The listing builds one solid part. Answer for the finished solid, in the listing's coordinates (mm). Coordinates: 2 decimals unless noted, no trailing zeros. Order: outer loops, then holes, each group sorted by start corner. A loop starts at its lowest first (then second) coordinate and runs counter-clockwise, first axis right, second up. Notation, with made-up numbers: (30, 76.5) - (69, 76.5) arc R26 cw to (69, 96.5) - close; hole circle Ø6 at (-17.75, -14). An arc over 180 degrees is marked (long way). Use one line per item in the form item = value. Start each with the question number.
Item 1: Consider line 1 along X through (y, z) = (2.4, -47); line 2 along Z through (x, y) = (50, 1.6); line 3 along Z through (x, y) = (59.5, 0.65). Determine where each line is inside the solid, lowest interval first. Write a range as [from, to].
Item 2: Each of these flat-tipped pins is pushed along its axis until it touches: pin 1 Ø1 at (x, y) = (59.5, 1.5) entering from +Z; pin 2 Ø1 at (y, z) = (1.5, -46) entering from +X; pin 3 Ø4.5 at (x, z) = (50.2, 92.2) entering from +Y (3 decimals); pin 4 Ø1.5 at (x, y) = (-71.5, 2) entering from -Z. Where does it stop, or does it pass through?
Item 3: Section C-C, the plane y = 1.6 is taken. Count the separate pieces of the cut face and the enclosed holes in it, and give its area (3 significant figures).
Item 4: Section B-B, the plane z = 51.5 is taken. Write down the section's boundary in (x, y) (3 decimals), and give its area (3 significant figures).
Item 5: Section A-A, the plane x = 0 is taken. Write down the section's boundary in (y, z) (3 decimals), and give its area (3 significant figures).
Item 6: Section D-D, the plane z = 24 is taken. Write down the section's boundary in (x, y) (3 decimals).
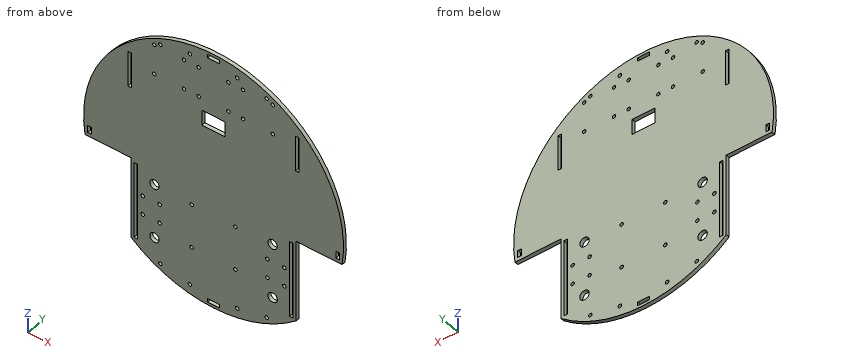
from build123d import *

# Parameters (mm, degrees)
SKETCH_1_R   = 1.5
SKETCH_1_R_2 = 4
SKETCH_1_R_3 = 1.45
SKETCH_1_W   = 10
SKETCH_1_H   = 3
SKETCH_1_W_2 = 19.6
SKETCH_1_H_2 = 12.9
SKETCH_1_W_3 = 3
SKETCH_1_H_3 = 6
SKETCH_1_H_4 = 65
SKETCH_1_H_5 = 30
BASE_DEPTH   = 3.175


with BuildPart() as part:
    # 草图1 → Base (new body)
    with BuildSketch(Plane(origin=(0, 0, 0), x_dir=(1, 0, 0), z_dir=(0, 1, 0))):
        with BuildLine():
            Line((-108.841874295, 15.92), (-70, 15.92))
            Line((-70, 15.92), (-70, 84.852813742))
            ThreePointArc((-70, 84.852813742), (0, 110), (70, 84.852813742))
            Line((70, 84.852813742), (70, 15.92))
            Line((70, 15.92), (108.841874295, 15.92))
            ThreePointArc((108.841874295, 15.92), (0, -110), (-108.841874295, 15.92))
        make_face()
        with Locations((-60, 43.92)):
            Circle(SKETCH_1_R, mode=Mode.SUBTRACT)
        with Locations((-60, 60)):
            Circle(SKETCH_1_R, mode=Mode.SUBTRACT)
        with Locations((-45.65, 60)):
            Circle(SKETCH_1_R, mode=Mode.SUBTRACT)
        with Locations((-45.65, 43.92)):
            Circle(SKETCH_1_R, mode=Mode.SUBTRACT)
        with Locations((60, 60)):
            Circle(SKETCH_1_R, mode=Mode.SUBTRACT)
        with Locations((45.65, 60)):
            Circle(SKETCH_1_R, mode=Mode.SUBTRACT)
        with Locations((45.65, 43.92)):
            Circle(SKETCH_1_R, mode=Mode.SUBTRACT)
        with Locations((60, 43.92)):
            Circle(SKETCH_1_R, mode=Mode.SUBTRACT)
        with Locations((-20, -100)):
            Circle(SKETCH_1_R, mode=Mode.SUBTRACT)
        with Locations((20, -100)):
            Circle(SKETCH_1_R, mode=Mode.SUBTRACT)
        with Locations((20, 100)):
            Circle(SKETCH_1_R, mode=Mode.SUBTRACT)
        with Locations((-20, 100)):
            Circle(SKETCH_1_R, mode=Mode.SUBTRACT)
        with Locations((-50, 75)):
            Circle(SKETCH_1_R_2, mode=Mode.SUBTRACT)
        with Locations((50, 75)):
            Circle(SKETCH_1_R_2, mode=Mode.SUBTRACT)
        with Locations((-18.5, 67)):
            Circle(SKETCH_1_R, mode=Mode.SUBTRACT)
        with Locations((-18.5, 30)):
            Circle(SKETCH_1_R, mode=Mode.SUBTRACT)
        with Locations((18.5, 30)):
            Circle(SKETCH_1_R, mode=Mode.SUBTRACT)
        with Locations((18.5, 67)):
            Circle(SKETCH_1_R, mode=Mode.SUBTRACT)
        with Locations((-12.6, -67)):
            Circle(SKETCH_1_R_3, mode=Mode.SUBTRACT)
        with Locations((-12.6, -92.2)):
            Circle(SKETCH_1_R_3, mode=Mode.SUBTRACT)
        with Locations((12.6, -92.2)):
            Circle(SKETCH_1_R_3, mode=Mode.SUBTRACT)
        with Locations((12.6, -67)):
            Circle(SKETCH_1_R_3, mode=Mode.SUBTRACT)
        with Locations((-45, 95)):
            Circle(SKETCH_1_R, mode=Mode.SUBTRACT)
        with Locations((45, 95)):
            Circle(SKETCH_1_R, mode=Mode.SUBTRACT)
        with Locations((45, -95)):
            Circle(SKETCH_1_R, mode=Mode.SUBTRACT)
        with Locations((-45, -95)):
            Circle(SKETCH_1_R, mode=Mode.SUBTRACT)
        with Locations((-50.2, -67)):
            Circle(SKETCH_1_R_3, mode=Mode.SUBTRACT)
        with Locations((-50.2, -92.2)):
            Circle(SKETCH_1_R_3, mode=Mode.SUBTRACT)
        with Locations((-25, -67)):
            Circle(SKETCH_1_R_3, mode=Mode.SUBTRACT)
        with Locations((-25, -92.2)):
            Circle(SKETCH_1_R_3, mode=Mode.SUBTRACT)
        with Locations((50.2, -92.2)):
            Circle(SKETCH_1_R_3, mode=Mode.SUBTRACT)
        with Locations((25, -92.2)):
            Circle(SKETCH_1_R_3, mode=Mode.SUBTRACT)
        with Locations((25, -67)):
            Circle(SKETCH_1_R_3, mode=Mode.SUBTRACT)
        with Locations((50.2, -67)):
            Circle(SKETCH_1_R_3, mode=Mode.SUBTRACT)
        with Locations((-50, 28.92)):
            Circle(SKETCH_1_R_2, mode=Mode.SUBTRACT)
        with Locations((50, 28.92)):
            Circle(SKETCH_1_R_2, mode=Mode.SUBTRACT)
        with Locations((0, -106)):
            Rectangle(SKETCH_1_W, SKETCH_1_H, mode=Mode.SUBTRACT)
        with Locations((0, -50)):
            Rectangle(SKETCH_1_W_2, SKETCH_1_H_2, mode=Mode.SUBTRACT)
        with Locations((0, 106)):
            Rectangle(SKETCH_1_W, SKETCH_1_H, mode=Mode.SUBTRACT)
        with Locations((105, 10)):
            Rectangle(SKETCH_1_W_3, SKETCH_1_H_3, mode=Mode.SUBTRACT)
        with Locations((-105, 10)):
            Rectangle(SKETCH_1_W_3, SKETCH_1_H_3, mode=Mode.SUBTRACT)
        with Locations((66, 51.352813742)):
            Rectangle(SKETCH_1_W_3, SKETCH_1_H_4, mode=Mode.SUBTRACT)
        with Locations((-66, 51.352813742)):
            Rectangle(SKETCH_1_W_3, SKETCH_1_H_4, mode=Mode.SUBTRACT)
        with Locations((71, -60)):
            Rectangle(SKETCH_1_W_3, SKETCH_1_H_5, mode=Mode.SUBTRACT)
        with Locations((-71, -60)):
            Rectangle(SKETCH_1_W_3, SKETCH_1_H_5, mode=Mode.SUBTRACT)
    extrude(amount=BASE_DEPTH)


solid = part.part
Response:
q1.line_1 = [-70, -67.5], [-64.5, 64.5], [67.5, 70]
q1.line_2 = [-97.98, -79], [-71, -32.92], [-24.92, 65.56], [68.44, 90.76], [93.64, 97.98]
q1.line_3 = [-92.52, -61.41], [-58.59, -45.33], [-42.51, 92.52]
q2.pin_1 = 92.84
q2.pin_2 = 70
q2.pin_3 = 3.175
q2.pin_4 = -15.92
q3.separate_pieces = 1
q3.enclosed_holes = 45
q3.area = 33,200 mm2
q4.outline = (-97.2, 0) - (-72.5, 0) - (-72.5, 3.175) - (-97.2, 3.175) - close; (-69.5, 0) - (-9.8, 0) - (-9.8, 3.175) - (-69.5, 3.175) - close; (9.8, 0) - (69.5, 0) - (69.5, 3.175) - (9.8, 3.175) - close; (72.5, 0) - (97.2, 0) - (97.2, 3.175) - (72.5, 3.175) - close
q4.area = 536 mm2
q5.outline = (0, -110) - (3.175, -110) - (3.175, -107.5) - (0, -107.5) - close; (0, -104.5) - (3.175, -104.5) - (3.175, 43.55) - (0, 43.55) - close; (0, 56.45) - (3.175, 56.45) - (3.175, 104.5) - (0, 104.5) - close; (0, 107.5) - (3.175, 107.5) - (3.175, 110) - (0, 110) - close
q5.area = 638 mm2
q6.outline = (-107.35, 0) - (107.35, 0) - (107.35, 3.175) - (-107.35, 3.175) - close
